For this review, take the finished solid that the model builds, in its own axes (mm). Round coordinates to 2 decimals unless told otherwise and drop trailing zeros. Loops run counter-clockwise (first coordinate to the right, second up) from the corner with the lowest first, then second, coordinate; pieces in that order, holes last. Notation, with made-up numbers: (6.5, -38.75) -> (48.5, -38.75) arc R17 ccw to (48.5, -8.75) -> close; hole circle Ø2 at (-1.75, 53.25). An arc over 180 degrees is marked (long way). One line per question, with ' | ' between items. Start each with the question number.
1. Consider section A-A (x = -12.5). Write out the cut boundary in (y, z).
2. Consider section D-D (y = 1.05). Count the separate pieces of the cut face and the enclosed holes in it, and give its area (3 significant figures).
3. Consider section C-C (z = -32.5). Write out the cut boundary in (x, y).
4. For pin 1 Ø0.8 at (x, y) = (87.5, 2) entering from -Z; pin 2 Ø0.9 at (y, z) = (2, -65) entering from -X; pin 3 Ø0.9 at (y, z) = (1, 80.5) entering from -X, all flat-tipped, find the tip position at first contact; note any pin that passes through.
5. Wall thickness on line 1 along Z through (x, y) = (-86.5, 2.2) (3 decimals); line 2 along Z through (x, y) = (-96, 2); line 3 along X through (y, z) = (0.6, 19.5): over which ranges is each line inside the solid? List them lowest first.
6. Consider section B-B (z = -11.5). Write out the cut boundary in (x, y).
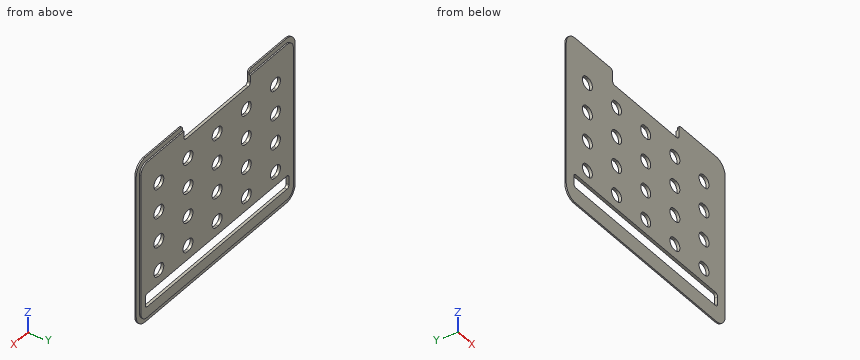
```python
from build123d import *

# Parameters (mm, degrees)
SKETCH1_W                = 240
SKETCH1_H                = 175
OUTER_PROFILE_DEPTH      = 1.5
SKETCH2_W                = 230
SKETCH2_H                = 165
INNER_PROFILE_DEPTH      = 1.5
FILLET1_R                = 9
FILLET2_R                = 13.5
CUTOUT_DEPTH             = 149.543764595
CUTOUTS_COUNT            = 3
CUTOUTS_PITCH            = 44
CUTOUTS_COUNT_DIR2       = 4
CUTOUTS_PITCH_DIR2       = 31
MIRROR1_COPY_1_DEPTH     = 149.543764595
MIRROR1_COPY_2_DEPTH     = 149.543764595
MIRROR1_COPY_3_DEPTH     = 149.543764595
MIRROR1_COPY_4_DEPTH     = 149.543764595
MIRROR1_COPY_5_DEPTH     = 149.543764595
MIRROR1_COPY_6_DEPTH     = 149.543764595
MIRROR1_COPY_7_DEPTH     = 149.543764595
MIRROR1_COPY_8_DEPTH     = 149.543764595
MIRROR1_COPY_9_DEPTH     = 149.543764595
MIRROR1_COPY_10_DEPTH    = 149.543764595
MIRROR1_COPY_11_DEPTH    = 149.543764595
MIRROR1_COPY_12_DEPTH    = 149.543764595
SKETCH4_W                = 217
SKETCH4_H                = 14
MESSAGE_WINDOW_DEPTH     = 149.543764595
MESSAGE_WINDOW_CORNERS_R = 3
SKETCH6_W                = 100
SKETCH6_H                = 15
BASE_CUTBACK_DEPTH       = 149.543764595
FILLET5_R                = 3


with BuildPart() as part:
    # Sketch1 → Outer Profile (new body)
    with BuildSketch(Plane(origin=(0, 0, 0), x_dir=(1, 0, 0), z_dir=(0, 1, 0))):
        Rectangle(SKETCH1_W, SKETCH1_H)
    extrude(amount=OUTER_PROFILE_DEPTH)

    # Sketch2 → Inner Profile (add)
    with BuildSketch(Plane(origin=(0, 1.5, 0), x_dir=(1, 0, 0), z_dir=(0, 1, 0))):
        Rectangle(SKETCH2_W, SKETCH2_H)
    extrude(amount=INNER_PROFILE_DEPTH)

    # Fillet1
    fillet1_edges = [part.edges().sort_by_distance(p)[0] for p in [
        (115, 2.25, 82.5),
        (115, 2.25, -82.5),
        (-115, 2.25, -82.5),
        (-115, 2.25, 82.5),
    ]]
    fillet(fillet1_edges, radius=FILLET1_R)

    # Fillet2
    fillet2_edges = [part.edges().sort_by_distance(p)[0] for p in [
        (120, 0.75, 87.5),
        (-120, 0.75, 87.5),
        (-120, 0.75, -87.5),
        (120, 0.75, -87.5),
    ]]
    fillet(fillet2_edges, radius=FILLET2_R)

    # Sketch3 → Cutout (cut, through all)
    with BuildSketch(Plane(origin=(0, 3, 0), x_dir=(1, 0, 0), z_dir=(0, 1, 0))):
        with BuildLine():
            Line((-1.25, -44.25), (1.25, -44.25))
            ThreePointArc((1.25, -44.25), (7.5, -50.5), (1.25, -56.75))
            Line((1.25, -56.75), (-1.25, -56.75))
            ThreePointArc((-1.25, -56.75), (-7.5, -50.5), (-1.25, -44.25))
        make_face()
    cutout = extrude(amount=-CUTOUT_DEPTH, mode=Mode.SUBTRACT)

    # Cutouts: Cutout 3 × 4
    with Locations(*[(-i * CUTOUTS_PITCH, 0, -j * CUTOUTS_PITCH_DIR2) for i in range(CUTOUTS_COUNT) for j in range(CUTOUTS_COUNT_DIR2) if (i, j) != (0, 0)]):
        add(cutout, mode=Mode.SUBTRACT)

    # Mirror1 copy 1 sketch → Mirror1 copy 1 (cut, through all)
    with BuildSketch(Plane(origin=(0, 3, -31), x_dir=(-1, 0, 0), z_dir=(0, 1, 0))):
        with BuildLine():
            Line((-1.25, 44.25), (1.25, 44.25))
            ThreePointArc((1.25, 44.25), (7.5, 50.5), (1.25, 56.75))
            Line((1.25, 56.75), (-1.25, 56.75))
            ThreePointArc((-1.25, 56.75), (-7.5, 50.5), (-1.25, 44.25))
        make_face()
    extrude(amount=-MIRROR1_COPY_1_DEPTH, mode=Mode.SUBTRACT)

    # Mirror1 copy 2 sketch → Mirror1 copy 2 (cut, through all)
    with BuildSketch(Plane(origin=(0, 3, -62), x_dir=(-1, 0, 0), z_dir=(0, 1, 0))):
        with BuildLine():
            Line((-1.25, 44.25), (1.25, 44.25))
            ThreePointArc((1.25, 44.25), (7.5, 50.5), (1.25, 56.75))
            Line((1.25, 56.75), (-1.25, 56.75))
            ThreePointArc((-1.25, 56.75), (-7.5, 50.5), (-1.25, 44.25))
        make_face()
    extrude(amount=-MIRROR1_COPY_2_DEPTH, mode=Mode.SUBTRACT)

    # Mirror1 copy 3 sketch → Mirror1 copy 3 (cut, through all)
    with BuildSketch(Plane(origin=(0, 3, -93), x_dir=(-1, 0, 0), z_dir=(0, 1, 0))):
        with BuildLine():
            Line((-1.25, 44.25), (1.25, 44.25))
            ThreePointArc((1.25, 44.25), (7.5, 50.5), (1.25, 56.75))
            Line((1.25, 56.75), (-1.25, 56.75))
            ThreePointArc((-1.25, 56.75), (-7.5, 50.5), (-1.25, 44.25))
        make_face()
    extrude(amount=-MIRROR1_COPY_3_DEPTH, mode=Mode.SUBTRACT)

    # Mirror1 copy 4 sketch → Mirror1 copy 4 (cut, through all)
    with BuildSketch(Plane(origin=(44, 3, 0), x_dir=(-1, 0, 0), z_dir=(0, 1, 0))):
        with BuildLine():
            Line((-1.25, 44.25), (1.25, 44.25))
            ThreePointArc((1.25, 44.25), (7.5, 50.5), (1.25, 56.75))
            Line((1.25, 56.75), (-1.25, 56.75))
            ThreePointArc((-1.25, 56.75), (-7.5, 50.5), (-1.25, 44.25))
        make_face()
    extrude(amount=-MIRROR1_COPY_4_DEPTH, mode=Mode.SUBTRACT)

    # Mirror1 copy 5 sketch → Mirror1 copy 5 (cut, through all)
    with BuildSketch(Plane(origin=(44, 3, -31), x_dir=(-1, 0, 0), z_dir=(0, 1, 0))):
        with BuildLine():
            Line((-1.25, 44.25), (1.25, 44.25))
            ThreePointArc((1.25, 44.25), (7.5, 50.5), (1.25, 56.75))
            Line((1.25, 56.75), (-1.25, 56.75))
            ThreePointArc((-1.25, 56.75), (-7.5, 50.5), (-1.25, 44.25))
        make_face()
    extrude(amount=-MIRROR1_COPY_5_DEPTH, mode=Mode.SUBTRACT)

    # Mirror1 copy 6 sketch → Mirror1 copy 6 (cut, through all)
    with BuildSketch(Plane(origin=(44, 3, -62), x_dir=(-1, 0, 0), z_dir=(0, 1, 0))):
        with BuildLine():
            Line((-1.25, 44.25), (1.25, 44.25))
            ThreePointArc((1.25, 44.25), (7.5, 50.5), (1.25, 56.75))
            Line((1.25, 56.75), (-1.25, 56.75))
            ThreePointArc((-1.25, 56.75), (-7.5, 50.5), (-1.25, 44.25))
        make_face()
    extrude(amount=-MIRROR1_COPY_6_DEPTH, mode=Mode.SUBTRACT)

    # Mirror1 copy 7 sketch → Mirror1 copy 7 (cut, through all)
    with BuildSketch(Plane(origin=(44, 3, -93), x_dir=(-1, 0, 0), z_dir=(0, 1, 0))):
        with BuildLine():
            Line((-1.25, 44.25), (1.25, 44.25))
            ThreePointArc((1.25, 44.25), (7.5, 50.5), (1.25, 56.75))
            Line((1.25, 56.75), (-1.25, 56.75))
            ThreePointArc((-1.25, 56.75), (-7.5, 50.5), (-1.25, 44.25))
        make_face()
    extrude(amount=-MIRROR1_COPY_7_DEPTH, mode=Mode.SUBTRACT)

    # Mirror1 copy 8 sketch → Mirror1 copy 8 (cut, through all)
    with BuildSketch(Plane(origin=(88, 3, 0), x_dir=(-1, 0, 0), z_dir=(0, 1, 0))):
        with BuildLine():
            Line((-1.25, 44.25), (1.25, 44.25))
            ThreePointArc((1.25, 44.25), (7.5, 50.5), (1.25, 56.75))
            Line((1.25, 56.75), (-1.25, 56.75))
            ThreePointArc((-1.25, 56.75), (-7.5, 50.5), (-1.25, 44.25))
        make_face()
    extrude(amount=-MIRROR1_COPY_8_DEPTH, mode=Mode.SUBTRACT)

    # Mirror1 copy 9 sketch → Mirror1 copy 9 (cut, through all)
    with BuildSketch(Plane(origin=(88, 3, -31), x_dir=(-1, 0, 0), z_dir=(0, 1, 0))):
        with BuildLine():
            Line((-1.25, 44.25), (1.25, 44.25))
            ThreePointArc((1.25, 44.25), (7.5, 50.5), (1.25, 56.75))
            Line((1.25, 56.75), (-1.25, 56.75))
            ThreePointArc((-1.25, 56.75), (-7.5, 50.5), (-1.25, 44.25))
        make_face()
    extrude(amount=-MIRROR1_COPY_9_DEPTH, mode=Mode.SUBTRACT)

    # Mirror1 copy 10 sketch → Mirror1 copy 10 (cut, through all)
    with BuildSketch(Plane(origin=(88, 3, -62), x_dir=(-1, 0, 0), z_dir=(0, 1, 0))):
        with BuildLine():
            Line((-1.25, 44.25), (1.25, 44.25))
            ThreePointArc((1.25, 44.25), (7.5, 50.5), (1.25, 56.75))
            Line((1.25, 56.75), (-1.25, 56.75))
            ThreePointArc((-1.25, 56.75), (-7.5, 50.5), (-1.25, 44.25))
        make_face()
    extrude(amount=-MIRROR1_COPY_10_DEPTH, mode=Mode.SUBTRACT)

    # Mirror1 copy 11 sketch → Mirror1 copy 11 (cut, through all)
    with BuildSketch(Plane(origin=(88, 3, -93), x_dir=(-1, 0, 0), z_dir=(0, 1, 0))):
        with BuildLine():
            Line((-1.25, 44.25), (1.25, 44.25))
            ThreePointArc((1.25, 44.25), (7.5, 50.5), (1.25, 56.75))
            Line((1.25, 56.75), (-1.25, 56.75))
            ThreePointArc((-1.25, 56.75), (-7.5, 50.5), (-1.25, 44.25))
        make_face()
    extrude(amount=-MIRROR1_COPY_11_DEPTH, mode=Mode.SUBTRACT)

    # Mirror1 copy 12 sketch → Mirror1 copy 12 (cut, through all)
    with BuildSketch(Plane(origin=(0, 3, 0), x_dir=(-1, 0, 0), z_dir=(0, 1, 0))):
        with BuildLine():
            Line((-1.25, 44.25), (1.25, 44.25))
            ThreePointArc((1.25, 44.25), (7.5, 50.5), (1.25, 56.75))
            Line((1.25, 56.75), (-1.25, 56.75))
            ThreePointArc((-1.25, 56.75), (-7.5, 50.5), (-1.25, 44.25))
        make_face()
    extrude(amount=-MIRROR1_COPY_12_DEPTH, mode=Mode.SUBTRACT)

    # Sketch4 → Message Window (cut, through all)
    with BuildSketch(Plane(origin=(0, 3, 0), x_dir=(1, 0, 0), z_dir=(0, 1, 0))):
        with Locations((0, 64.25)):
            Rectangle(SKETCH4_W, SKETCH4_H)
    extrude(amount=-MESSAGE_WINDOW_DEPTH, mode=Mode.SUBTRACT)

    # Message Window Corners
    message_window_corners_edges = [part.edges().sort_by_distance(p)[0] for p in [
        (-108.5, 1.5, -57.25),
        (-108.5, 1.5, -71.25),
        (108.5, 1.5, -71.25),
        (108.5, 1.5, -57.25),
    ]]
    fillet(message_window_corners_edges, radius=MESSAGE_WINDOW_CORNERS_R)

    # Sketch6 → Base Cutback (cut, through all)
    with BuildSketch(Plane(origin=(0, 3, 0), x_dir=(1, 0, 0), z_dir=(0, 1, 0))):
        with Locations((0, -80)):
            Rectangle(SKETCH6_W, SKETCH6_H)
    extrude(amount=-BASE_CUTBACK_DEPTH, mode=Mode.SUBTRACT)

    # Fillet5
    fillet5_edges = [part.edges().sort_by_distance(p)[0] for p in [
        (50, 0.75, 87.5),
        (50, 1.5, 72.5),
        (-50, 0.75, 87.5),
        (-50, 1.5, 72.5),
    ]]
    fillet(fillet5_edges, radius=FILLET5_R)


solid = part.part
```
Answer block:
1) outline: (0, -87.5) -> (1.5, -87.5) -> (1.5, -82.5) -> (3, -82.5) -> (3, -71.25) -> (0, -71.25) -> close; (0, -57.25) -> (3, -57.25) -> (3, 72.5) -> (0, 72.5) -> close
2) separate pieces: 1 | enclosed holes: 21 | area: 34,200 mm2
3) outline: (-120, 0) -> (120, 0) -> (120, 1.5) -> (115, 1.5) -> (115, 3) -> (-115, 3) -> (-115, 1.5) -> (-120, 1.5) -> close
4) pin 1: stops at z = -82.5 | pin 2: stops at x = -115 | pin 3: stops at x = -118.57
5) line 1: z = -82.5 to -71.25, -57.25 to -48.745, -36.255 to -17.745, -5.255 to 13.255, 25.745 to 44.255, 56.745 to 82.5 | line 2: z = -82.5 to -71.25, -57.25 to 82.5 | line 3: x = -120 to -95.5, -80.5 to -51.5, -36.5 to -7.5, 7.5 to 36.5, 51.5 to 80.5, 95.5 to 120
6) outline: (-120, 0) -> (-95.5, 0) -> (-95.5, 3) -> (-115, 3) -> (-115, 1.5) -> (-120, 1.5) -> close; (-80.5, 0) -> (-51.5, 0) -> (-51.5, 3) -> (-80.5, 3) -> close; (-36.5, 0) -> (-7.5, 0) -> (-7.5, 3) -> (-36.5, 3) -> close; (7.5, 0) -> (36.5, 0) -> (36.5, 3) -> (7.5, 3) -> close; (51.5, 0) -> (80.5, 0) -> (80.5, 3) -> (51.5, 3) -> close; (95.5, 0) -> (120, 0) -> (120, 1.5) -> (115, 1.5) -> (115, 3) -> (95.5, 3) -> close
